from build123d import *

# Parameters (mm, degrees)
CROQUIS1_R                   = 13
SALIENTE_EXTRUIR1_DEPTH      = 2.4
CROQUIS2_R                   = 10
SALIENTE_EXTRUIR2_DEPTH      = 183.48
SALIENTE_EXTRUIR3_DEPTH      = 10
SALIENTE_EXTRUIR3_DEPTH_BACK = 10
CROQUIS3_R                   = 5


with BuildPart() as part:
    # Croquis1 → Saliente-Extruir1 (new body)
    with BuildSketch(Plane(origin=(0, 0, 0), x_dir=(1, 0, 0), z_dir=(0, 1, 0))):
        with Locations(Location((0, 0, 0), (0, 0, 270))):
            Circle(CROQUIS1_R)
    extrude(amount=SALIENTE_EXTRUIR1_DEPTH)

    # Croquis2 → Saliente-Extruir2 (add)
    with BuildSketch(Plane.XZ):
        with Locations(Location((0, 0, 0), (0, 0, 270))):
            Circle(CROQUIS2_R)
    extrude(amount=SALIENTE_EXTRUIR2_DEPTH)

    # Croquis3 → Saliente-Extruir3 (add, two sides: drawn at the far end of the back side and taken through both)
    with BuildSketch(Plane(origin=(0, 0, 0), x_dir=(0, 0, -1), z_dir=(1, 0, 0)).offset(-SALIENTE_EXTRUIR3_DEPTH_BACK)):
        with BuildLine():
            Line((-12, -183.48), (12, -183.48))
            ThreePointArc((12, -183.48), (0, -195.48), (-12, -183.48))
        make_face()
        with Locations((0, -189.48)):
            Circle(CROQUIS3_R, mode=Mode.SUBTRACT)
    extrude(amount=SALIENTE_EXTRUIR3_DEPTH + SALIENTE_EXTRUIR3_DEPTH_BACK)


solid = part.part
Could you check a few things on this model? Use its own coordinates, in mm. A direction names the side the tool comes from. Coordinates: 2 decimals unless noted, no trailing zeros. Order: outer loops, then holes, each group sorted by start corner. A loop starts at its lowest first (then second) coordinate and runs counter-clockwise, first axis right, second up. Notation, with made-up numbers: (-28, 15) - (0, 15) arc R29 cw to (0, 40) - close; hole circle Ø5 at (50.25, -38). An arc over 180 degrees is marked (long way). Answer in a Markdown table with one row per item. Add a question column.
(1) I need wall thicknesses on L1, parallel to Y at x = 3.75, z = 0; L2, parallel to X at y = -125.5, z = -0.75; L3, parallel to Z at x = 0, y = -155. Which ranges of each line are inside material? Lowest first, please.
(2) If we section it at A-A, the plane z = -2: Please give me the cut outline in (x, y), then the cut area to 3 significant figures.
(3) If we section it at C-C, the plane y = -189.48: Please give me the cut outline in (x, z), then the cut area to 3 significant figures.
(4) On a 3-axis mill with a long thin cutter (end or side, diameter ignored), from which of +Z, -Z, +X, -X, +Y, -Y can I reach the whole of each face in a straight line? I mean faces 1 (the face through (0, -183.48, 10.5)), 2 (the face through (-9.76, -90.46, 2.17)), 3 (the face through (10, -184, 0)). Say none if no direction works.
(5) If we mould it in two halves opening along Y, with no side actions, what happens to faces 4 (the face through (-0.14, -195.477, -0.264)), 5 (the face through (-10, -184, 0)), 6 (the face through (-8, 0, 7))? For each: released by +Y, released by -Y, zero draft, split by the parting line, or undercut.
(6) If we section it at B-B, the plane x = -7.5: Please give me the cut outline in (y, z).
(7) Will these pins go through, and if not, where does the flat tip stop? pin 1 (1.5 mm diameter, centred on x = 2, z = -9.5, fed in from -Y); pin 2 (1.5 mm diameter, centred on y = -43.5, z = -0.5, fed in from -X); pin 3 (8 mm diameter, centred on y = -135.5, z = 7, fed in from -X).
(8) If we section it at D-D, the plane x = 5.25: Please give me the cut outline in (y, z).
Results are:
| question | item | result |
|---|---|---|
| 1 | L1 | y = -195.48 to -194.48, -184.48 to 2.4 |
| 1 | L2 | x = -9.97 to 9.97 |
| 1 | L3 | z = -10 to 10 |
| 2 | outline | (-12.85, 0) - (-9.8, 0) - (-9.8, -183.48) - (-10, -183.48) - (-10, -184.9) - (10, -184.9) - (10, -183.48) - (9.8, -183.48) - (9.8, 0) - (12.85, 0) - (12.85, 2.4) - (-12.85, 2.4) - close; (-10, -195.31) - (10, -195.31) - (10, -194.06) - (-10, -194.06) - close |
| 2 | area | 3,710 mm2 |
| 3 | outline | (-10, -10.39) - (10, -10.39) - (10, -5) - (-10, -5) - close; (-10, 5) - (10, 5) - (10, 10.39) - (-10, 10.39) - close |
| 3 | area | 216 mm2 |
| 4 | face 1 | +Z |
| 4 | face 2 | none |
| 4 | face 3 | +Z, -Z, +X, -Y |
| 5 | face 4 | released by -Y |
| 5 | face 5 | zero draft |
| 5 | face 6 | undercut |
| 6 | outline | (-183.48, -12) - (-183.48, -6.61) - (0, -6.61) - (0, -10.62) - (2.4, -10.62) - (2.4, 10.62) - (0, 10.62) - (0, 6.61) - (-183.48, 6.61) - (-183.48, 12) arc R12 ccw to start; hole circle Ø10 at (-189.48, 0) |
| 7 | pin 1 | stops at y = -191.69 |
| 7 | pin 2 | stops at x = -10 |
| 7 | pin 3 | stops at x = -9.54 |
| 8 | outline | (-183.48, -12) - (-183.48, -8.51) - (0, -8.51) - (0, -11.89) - (2.4, -11.89) - (2.4, 11.89) - (0, 11.89) - (0, 8.51) - (-183.48, 8.51) - (-183.48, 12) arc R12 ccw to start; hole circle Ø10 at (-189.48, 0) |
